The figure shows three views and two pictorial views of one solid part (mm, origin at its lowest corner). Answer the questions. Coordinates: 2 decimals unless noted, no trailing zeros. Loops run counter-clockwise (first coordinate to the right, second up) from the corner with the lowest first, then second, coordinate; pieces in that order, holes last.
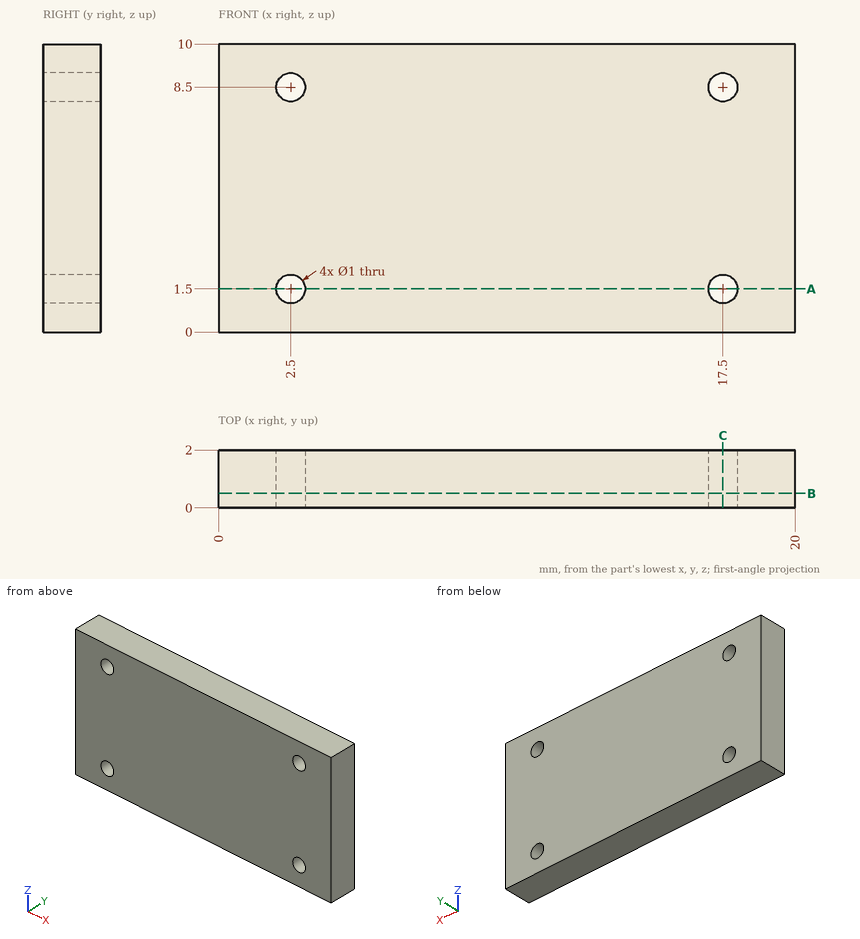
1. A cutting plane is placed at B-B, the plane y = 0.5. Give the vertices of the cut face in (x, z), then the cut area to 3 significant figures.
2. A cutting plane is placed at C-C, the plane x = 17.5. Give the vertices of the cut face in (y, z), then the cut area to 3 significant figures.
3. A cutting plane is placed at A-A, the plane z = 1.5. Give the vertices of the cut face in (x, y), then the cut area to 3 significant figures.
4. Straight lines are drawn through the part: probe 1 along Z at (x, y) = (2.5, 1); probe 2 along Z at (x, y) = (17.25, 0.35); probe 3 along X at (y, z) = (1.65, 8.75). For each, find the intervals that lie inside material, in ascending order.
Answers below:
1. outline: (0, 0) - (20, 0) - (20, 10) - (0, 10) - close; hole circle Ø1 at (2.5, 1.5); hole circle Ø1 at (2.5, 8.5); hole circle Ø1 at (17.5, 1.5); hole circle Ø1 at (17.5, 8.5)
1. area: 197 mm2
2. outline: (0, 0) - (2, 0) - (2, 1) - (0, 1) - close; (0, 2) - (2, 2) - (2, 8) - (0, 8) - close; (0, 9) - (2, 9) - (2, 10) - (0, 10) - close
2. area: 16.0 mm2
3. outline: (0, 0) - (2, 0) - (2, 2) - (0, 2) - close; (3, 0) - (17, 0) - (17, 2) - (3, 2) - close; (18, 0) - (20, 0) - (20, 2) - (18, 2) - close
3. area: 36.0 mm2
4. probe 1: z = 0 to 1, 2 to 8, 9 to 10
4. probe 2: z = 0 to 1.07, 1.93 to 8.07, 8.93 to 10
4. probe 3: x = 0 to 2.07, 2.93 to 17.07, 17.93 to 20
